```python
from build123d import *

# Parameters (mm, degrees)
F0_W     = 94.2402782384
F0_H     = 118.9312338829
F1_DEPTH = 63.5
F2_SIZE  = 25.4
F3_R     = 6.35
F4_R     = 2.54
F5_R     = 12.7
F6_R     = 2.54
F7_W     = 89.1602782384
F7_H     = 30.6605122421
F8_DEPTH = 1.27


with BuildPart() as f1:
    # F0 (on Front) → F1 (new body)
    with BuildSketch(Plane.XZ):
        with Locations((1.3193635968, 0)):
            Rectangle(F0_W, F0_H)
    extrude(amount=F1_DEPTH)

    # F2
    f2_edges = [f1.edges().sort_by_distance(p)[0] for p in [
        (1.319364, -63.5, 59.465617),
    ]]
    chamfer(f2_edges, length=F2_SIZE)

    # F3
    f3_edges = [f1.edges().sort_by_distance(p)[0] for p in [
        (1.319364, -63.5, 34.065617),
        (1.319364, -38.1, 59.465617),
    ]]
    fillet(f3_edges, radius=F3_R)

    # F4
    f4_edges = [f1.edges().sort_by_distance(p)[0] for p in [
        (-45.800776, -17.734872, 59.465617),
        (-45.800776, -50.8, 46.765617),
        (-45.800776, -63.5, -14.015128),
        (-45.800776, -63.016635, 33.865401),
        (-45.800776, -37.899784, 58.982252),
        (48.439503, -17.734872, 59.465617),
        (48.439503, -37.899784, 58.982252),
        (48.439503, -50.8, 46.765617),
        (48.439503, -63.016635, 33.865401),
        (48.439503, -63.5, -14.015128),
    ]]
    fillet(f4_edges, radius=F4_R)

    # F5
    f5_edges = [f1.edges().sort_by_distance(p)[0] for p in [
        (1.319364, 0, -59.465617),
    ]]
    fillet(f5_edges, radius=F5_R)

    # F6
    f6_edges = [f1.edges().sort_by_distance(p)[0] for p in [
        (48.439503, 0, 5.08),
        (48.439503, -3.719744, -55.745873),
        (-45.800776, 0, 5.08),
        (-45.800776, -3.719744, -55.745873),
    ]]
    fillet(f6_edges, radius=F6_R)

    # F7 (on face) → F8 (join)
    with BuildSketch(Plane(origin=(0, -48.7828084707, 48.7828084707), x_dir=(1, 0, 0), z_dir=(0, -0.7071067812, 0.7071067812))):
        with Locations((1.3193635968, -2.8527396186)):
            Rectangle(F7_W, F7_H)
    extrude(amount=F8_DEPTH)


solid = f1.part
```
Part model, mm, in its own coordinate system. A direction names the side the tool comes from. Coordinates: 2 decimals unless noted, no trailing zeros. Write each loop counter-clockwise with the first axis right and the second up, starting at its lowest first coordinate (ties: lowest second). Pieces come first, ordered by that corner, then holes.
Item 1: Mould opens along Y. For faces 4 (the face through (1.943, -3.622, -55.647)), 5 (the face through (1.943, -37.867, 58.996)), 6 (the face through (-45.08, -50.41, 46.07)), 7 (the face through (1, -36, -59.466)) say: released by +Y, released by -Y, zero draft, split by the parting line, or undercut.
Item 2: Probe line 1 (Z direction, x = -12.5, y = -7.5); line 2 (Z direction, x = 34.5, y = -58); line 3 (Y direction, x = -30.5, z = 52). List the from-to ranges inside material, lowest first.
Item 3: Pin check, flat tip, straight feed: pin 1 (12 mm diameter, centred on x = 28, y = -6.5, fed in from -Z). Stop position of the tip, or through.
Item 4: Slice it at A-A (x = -32.5). Write the cut outline in (y, z), and give its area (3 significant figures).
Item 5: Which spindle directions (+Z, -Z, +X, -X, +Y, -Y) get a long thin tool onto all of the face, cutting with end or side? Do faces 1 (the face through (1.943, -63.003, 33.898)), 2 (the face through (45.9, -51, 47)), 3 (the face through (-45.801, -31, -1)). Say none if no direction does.
Results found:
1. face 4: released by +Y
1. face 5: undercut
1. face 6: released by -Y
1. face 7: zero draft
2. line 1: z = -58.35 to 59.47
2. line 2: z = -59.47 to 41.36
2. line 3: y = -47.36 to 0
3. pin 1: stops at z = -59.46
4. outline: (-63.5, -56.93) arc R2.54 ccw to (-60.96, -59.47) - (-12.7, -59.47) arc R12.7 ccw to (0, -46.77) - (0, 56.93) arc R2.54 ccw to (-2.54, 59.47) - (-35.47, 59.47) arc R6.35 ccw to (-39.96, 57.61) - (-40.86, 58.5) - (-62.54, 36.82) - (-61.64, 35.93) arc R6.35 ccw to (-63.5, 31.44) - close
4. area: 7,230 mm2
5. face 1: +X, -X, -Y
5. face 2: +Z, +X, -Y
5. face 3: +Z, -Z, -X, +Y, -Y
